```python
from build123d import *


with BuildPart() as f1:
    # F0 (on Front) → F1 (revolve)
    with BuildSketch(Plane.XZ):
        with BuildLine():
            Line((0, 0), (15.367, 0))
            Line((15.367, 0), (15.748, 0.635))
            Line((15.748, 0.635), (15.748, 5.08))
            ThreePointArc((15.748, 5.08), (15.45042, 5.79842), (14.732, 6.096))
            Line((14.732, 6.096), (12.446, 6.096))
            Line((12.446, 6.096), (10.668, 9.398))
            Line((10.668, 9.398), (12.446, 12.7))
            Line((12.446, 12.7), (2.286, 12.7))
            ThreePointArc((2.286, 12.7), (2.816039, 15.7737), (2.286, 18.8474))
            Line((2.286, 18.8474), (4.489498, 18.8474))
            ThreePointArc((4.489498, 18.8474), (2.205484, 22.156792), (1.401251, 26.09659))
            Line((1.401251, 26.09659), (1.401251, 56.192838))
            Line((1.401251, 56.192838), (3.532426, 56.192838))
            Line((3.532426, 56.192838), (0.475527, 63.946038))
            ThreePointArc((0.475527, 63.946038), (0.982077, 65.084624), (0, 65.85176))
            Line((0, 65.85176), (0, 0))
        make_face()
    revolve(axis=Axis((0, 0, 32.92588), (0, 0, -1)))


solid = f1.part
```
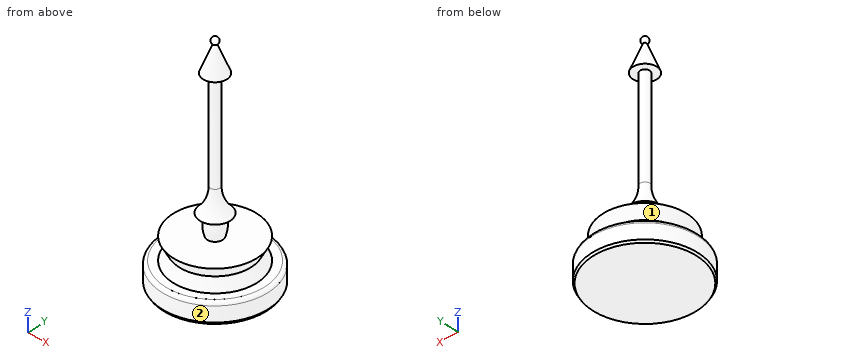
Source: CAD feature listing. Evaluate the final solid. Frame: model axes, mm. Face numbers are marked on the shaded views. A direction names the side the tool comes from. Round coordinates to 2 decimals unless told otherwise and drop trailing zeros. Write each loop counter-clockwise with the first axis right and the second up, starting at its lowest first coordinate (ties: lowest second). Pieces come first, ordered by that corner, then holes. Notation, with made-up numbers: M -26,-12.75 L 4,-12.75 A27 ccw 4,20.25 Z; hole C 19.25,51 d10. An arc over 180 degrees is marked long. Answer as a JSON object with one key per item and string values. Group by question number.
(1) Reachability of the marked faces 1 and 2 from +Z, -Z, +X, -X, +Y, -Y: full face, straight path, thin tool, end or side. Return the list, or none.
(2) First-contact query: pin 1 (1 mm diameter, centred on x = -0.5, y = -12.5, fed in from -Z); pin 2 (12 mm diameter, centred on x = -4, z = 33, fed in from +Y); pin 3 (1.5 mm diameter, centred on x = -10, y = 12.5, fed in from +Z); pin 4 (1 mm diameter, centred on x = -2.5, z = 21.5, fed in from +Y). Flat tips, straight axial feed; report the tip coordinate or a pass-through.
(3) Ray query, line 1 (Z direction, x = -12.5, y = 4.5); line 2 (Z direction, x = 3, y = -10); line 3 (Z direction, x = 2, y = 11.5). Return the intervals inside material, ascending. Write a range as [from, to].
(4) Section query A-A on z = 50. Output: boundary loops of the cut face in (x, y).
Computed values:
{
 "1": {"face 1": "none", "face 2": "+Z, -Z"},
 "2": {"pin 1": "z = 0", "pin 2": "y = 1.4", "pin 3": "z = 5.95", "pin 4": "y = 1.66"},
 "3": {"line 1": "[0, 6.1]", "line 2": "[0, 12.7]", "line 3": "[0, 7.53], [11.26, 12.7]"},
 "4": {"outline": "C 0,0 d2.8"}
}
